CAD build for the part. Positions are in the model's coordinates, mm. Coordinates: 2 decimals unless noted, no trailing zeros. Order: outer loops, then holes, each group sorted by start corner. A loop starts at its lowest first (then second) coordinate and runs counter-clockwise, first axis right, second up. Notation, with made-up numbers: M 42,79 L 54,79 A19 ccw 54,83 Z; hole C 36.25,46.25 d2. An arc over 180 degrees is marked long. Write item = value, one per line. Start each with the question number.
```python
from build123d import *

# Parameters (mm, degrees)
SKETCH1_R               = 100
BOSS_EXTRUDE1_DEPTH     = 10
FILL_PATTERN1_OUTLINE_R = 4
FILL_PATTERN1_DEPTH     = 10


# Read off the part's stored shape, not the designer's step: Fill Pattern1
with BuildPart() as part:
    # Sketch1 → Boss-Extrude1 (new body)
    with BuildSketch(Plane.XY):
        Circle(SKETCH1_R)
    extrude(amount=BOSS_EXTRUDE1_DEPTH)

    # Fill Pattern1 outline → Fill Pattern1 (cut)
    with BuildSketch(Plane.XY):
        with Locations((-44.09081537, 25.455844123)):
            Circle(FILL_PATTERN1_OUTLINE_R)
        with Locations((0, 50.911688245)):
            Circle(FILL_PATTERN1_OUTLINE_R)
        with Locations((-14.696938457, 42.426406871)):
            Circle(FILL_PATTERN1_OUTLINE_R)
        with Locations((-29.393876913, 33.941125497)):
            Circle(FILL_PATTERN1_OUTLINE_R)
        with Locations((-29.393876913, 16.970562748)):
            Circle(FILL_PATTERN1_OUTLINE_R)
        with Locations((-44.09081537, 8.485281374)):
            Circle(FILL_PATTERN1_OUTLINE_R)
        with Locations((-44.09081537, -8.485281374)):
            Circle(FILL_PATTERN1_OUTLINE_R)
        with Locations((-44.09081537, -25.455844123)):
            Circle(FILL_PATTERN1_OUTLINE_R)
        with Locations((14.696938457, 42.426406871)):
            Circle(FILL_PATTERN1_OUTLINE_R)
        with Locations((0, 33.941125497)):
            Circle(FILL_PATTERN1_OUTLINE_R)
        with Locations((-14.696938457, 25.455844123)):
            Circle(FILL_PATTERN1_OUTLINE_R)
        with Locations((-14.696938457, 8.485281374)):
            Circle(FILL_PATTERN1_OUTLINE_R)
        with Locations((-29.393876913, 0)):
            Circle(FILL_PATTERN1_OUTLINE_R)
        with Locations((-29.393876913, -16.970562748)):
            Circle(FILL_PATTERN1_OUTLINE_R)
        with Locations((-29.393876913, -33.941125497)):
            Circle(FILL_PATTERN1_OUTLINE_R)
        with Locations((29.393876913, 33.941125497)):
            Circle(FILL_PATTERN1_OUTLINE_R)
        with Locations((14.696938457, 25.455844123)):
            Circle(FILL_PATTERN1_OUTLINE_R)
        with Locations((0, 16.970562748)):
            Circle(FILL_PATTERN1_OUTLINE_R)
        Circle(FILL_PATTERN1_OUTLINE_R)
        with Locations((-14.696938457, -8.485281374)):
            Circle(FILL_PATTERN1_OUTLINE_R)
        with Locations((-14.696938457, -25.455844123)):
            Circle(FILL_PATTERN1_OUTLINE_R)
        with Locations((-14.696938457, -42.426406871)):
            Circle(FILL_PATTERN1_OUTLINE_R)
        with Locations((44.09081537, 25.455844123)):
            Circle(FILL_PATTERN1_OUTLINE_R)
        with Locations((29.393876913, 16.970562748)):
            Circle(FILL_PATTERN1_OUTLINE_R)
        with Locations((14.696938457, 8.485281374)):
            Circle(FILL_PATTERN1_OUTLINE_R)
        with Locations((14.696938457, -8.485281374)):
            Circle(FILL_PATTERN1_OUTLINE_R)
        with Locations((0, -16.970562748)):
            Circle(FILL_PATTERN1_OUTLINE_R)
        with Locations((0, -33.941125497)):
            Circle(FILL_PATTERN1_OUTLINE_R)
        with Locations((0, -50.911688245)):
            Circle(FILL_PATTERN1_OUTLINE_R)
        with Locations((44.09081537, 8.485281374)):
            Circle(FILL_PATTERN1_OUTLINE_R)
        with Locations((29.393876913, 0)):
            Circle(FILL_PATTERN1_OUTLINE_R)
        with Locations((29.393876913, -16.970562748)):
            Circle(FILL_PATTERN1_OUTLINE_R)
        with Locations((14.696938457, -25.455844123)):
            Circle(FILL_PATTERN1_OUTLINE_R)
        with Locations((14.696938457, -42.426406871)):
            Circle(FILL_PATTERN1_OUTLINE_R)
        with Locations((44.09081537, -8.485281374)):
            Circle(FILL_PATTERN1_OUTLINE_R)
        with Locations((44.09081537, -25.455844123)):
            Circle(FILL_PATTERN1_OUTLINE_R)
        with Locations((29.393876913, -33.941125497)):
            Circle(FILL_PATTERN1_OUTLINE_R)
    extrude(amount=FILL_PATTERN1_DEPTH, mode=Mode.SUBTRACT)


solid = part.part
```
1. Probe L1, parallel to Y at x = -46, z = 6.75; L2, parallel to X at y = 26, z = 8.5; L3, parallel to X at y = 43.5, z = 3. List the from-to ranges inside material, lowest first.
2. Flat gauge pins, fed straight in: pin 1 (5 mm diameter, centred on x = 29.39, y = -16.97, fed in from -Z); pin 2 (4 mm diameter, centred on y = -40, z = 3.5, fed in from +X); pin 3 (3 mm diameter, centred on x = -30.5, z = 6, fed in from -Y); pin 4 (3 mm diameter, centred on y = 12.5, z = 1, fed in from -X). Where does each tip first touch, or does it go through?
3. Mould opens along Y. For faces 1 (the flat face through (-1, -21, 10)), 2 (the cylindrical face through (-0.867, 47.007, 4.93)) say: released by +Y, released by -Y, zero draft, split by the parting line, or undercut.
4. Slice it at B-B (y = 0). Write the cut outline in (x, z), plus the area to 3 significant figures.
5. Slice it at A-A (x = 0). Give the number of separate pieces and of enclosed holes in the cut face, plus the area to 3 significant figures.
6. Slice it at C-C (x = 81). Write the cut outline in (y, z).
Calculated:
q1.L1 = -88.79 to -28.97, -21.94 to -12, -4.97 to 4.97, 12 to 21.94, 28.97 to 88.79
q1.L2 = -96.56 to -48.05, -40.13 to -18.66, -10.73 to 10.73, 18.66 to 40.13, 48.05 to 96.56
q1.L3 = -90.04 to -18.55, -10.84 to 10.84, 18.55 to 90.04
q2.pin_1 = through
q2.pin_2 = 92.5
q2.pin_3 = -95.7
q2.pin_4 = -99.39
q3.face_1 = zero draft
q3.face_2 = undercut
q4.outline = M -100,0 L -33.39,0 L -33.39,10 L -100,10 Z; M -25.39,0 L -4,0 L -4,10 L -25.39,10 Z; M 4,0 L 25.39,0 L 25.39,10 L 4,10 Z; M 33.39,0 L 100,0 L 100,10 L 33.39,10 Z
q4.area = 1,760 mm²
q5.separate_pieces = 8
q5.enclosed_holes = 0
q5.area = 1,440 mm²
q6.outline = M -58.64,0 L 58.64,0 L 58.64,10 L -58.64,10 Z
